Build history of the part. All positions in model axes, mm. A direction names the side the tool comes from. Give positions to 0.01 mm unless a question says otherwise; leave off trailing zeros. Order: outer loops, then holes, each group sorted by start corner. A loop starts at its lowest first (then second) coordinate and runs counter-clockwise, first axis right, second up. Notation, with made-up numbers: M -11.75,-26 L 7.25,-26 A21 ccw 7.25,-13 Z; hole C -4,84 d5. An arc over 180 degrees is marked long. One line per item, written item: value.
from build123d import *

# Parameters (mm, degrees)
F0_W           = 200
F0_H           = 200
F1_DEPTH       = 200
F2_W           = 160
F2_H           = 130
F3_DEPTH       = 160
F5_DEPTH       = 24
F7_R           = 5
F8_DEPTH       = 25
F9_DEPTH       = 25
F9_DEPTH_BACK  = 203.2
F10_DEPTH      = 25
F10_DEPTH_BACK = 215.8


with BuildPart() as f1:
    # F0 (on Top) → F1 (new body)
    with BuildSketch(Plane.XY):
        Rectangle(F0_W, F0_H)
    extrude(amount=F1_DEPTH)

    # F2 (on face) → F3 (cut)
    with BuildSketch(Plane.XZ.offset(100)):
        with Locations((0, 80)):
            Rectangle(F2_W, F2_H)
    extrude(amount=-F3_DEPTH, mode=Mode.SUBTRACT)

    # F4 (on face) → F5 (cut)
    with BuildSketch(Plane.YZ.offset(100)):
        Polygon((-7.5, 67.5), (0, 67.5), (7.5, 67.5), (7.5, 82.5), (-7.5, 82.5), align=None)
    extrude(amount=-F5_DEPTH, mode=Mode.SUBTRACT)

    # F6 (on face) + F7 (on face) → F8 (cut)
    with BuildSketch(Plane(origin=(-100, 0, 0), x_dir=(0, -1, 0), z_dir=(-1, 0, 0))):
        Polygon((-7.5, 67.5), (0, 67.5), (7.5, 67.5), (7.5, 82.5), (-7.5, 82.5), align=None)
    with BuildSketch(Plane.YZ.offset(100)):
        with Locations((70, 9)):
            Circle(F7_R)
        with Locations((-70, 9)):
            Circle(F7_R)
    extrude(amount=-F8_DEPTH, mode=Mode.SUBTRACT)

    # F7 (on face) → F9 (cut, two sides)
    with BuildSketch(Plane.YZ.offset(100)) as f9_sk:
        with Locations((-70, 9)):
            Circle(F7_R)
    extrude(amount=F9_DEPTH, mode=Mode.SUBTRACT)
    extrude(f9_sk.sketch, amount=-F9_DEPTH_BACK, mode=Mode.SUBTRACT)

    # F7 (on face) → F10 (cut, two sides)
    with BuildSketch(Plane.YZ.offset(100)) as f10_sk:
        with Locations((70, 9)):
            Circle(F7_R)
    extrude(amount=F10_DEPTH, mode=Mode.SUBTRACT)
    extrude(f10_sk.sketch, amount=-F10_DEPTH_BACK, mode=Mode.SUBTRACT)


solid = f1.part
1) Saw through at C-C, the plane x = 15.5. Write the cut outline in (y, z), then the cut area to 3 significant figures.
Check values:
outline: M -100,0 L 100,0 L 100,200 L -100,200 L -100,145 L 60,145 L 60,15 L -100,15 Z; hole C -70,9 d10; hole C 70,9 d10
area: 19,000 mm^2
2) Saw through at B-B, the plane z = 9. Write the cut outline in (x, y).
Check values:
outline: M -100,-100 L 100,-100 L 100,-75 L -100,-75 Z; M -100,-65 L 100,-65 L 100,65 L -100,65 Z; M -100,75 L 100,75 L 100,100 L -100,100 Z
3) Drill centre lines: probe 1 along Z at (x, y) = (-3.5, -70); probe 2 along X at (y, z) = (31, 111.5); probe 3 along Z at (x, y) = (-42, 70). Where is each one in solid material? Low to high. Write a range as from..to.
Check values:
probe 1: 0..4, 14..15, 145..200
probe 2: -100..-80, 80..100
probe 3: 0..4, 14..200
4) Saw through at D-D, the plane y = 48.5. Write the cut outline in (x, z).
Check values:
outline: M -100,0 L 100,0 L 100,200 L -100,200 Z; hole M -80,15 L 80,15 L 80,145 L -80,145 Z
5) Mould opens along Z. For faces 1 (the face through (-1, 1, 0)), 2 (the face through (-100, -1, 99)), 3 (the face through (-90, 0, 67.5)) say: released by +Z, released by -Z, zero draft, split by the parting line, or undercut.
Check values:
face 1: released by -Z
face 2: zero draft
face 3: undercut
6) Tool access for faces 4 (the face through (-1, 100, 99)), 5 (the face through (-1, -21, 15)), 6 (the face through (-90, -7.5, 75)): list every direction of +Z, -Z, +X, -X, +Y, -Y with a clear straight run to the whole face (end or side of a thin tool).
Check values:
face 4: +Z, -Z, +X, -X, +Y
face 5: -Y
face 6: +X, -X
7) Saw through at A-A, the plane y = -70. Write the cut outline in (x, z), then the cut area to 3 significant figures.
Check values:
outline: M -100,0 L 100,0 L 100,4 L -100,4 Z; M -100,14 L 100,14 L 100,200 L -100,200 Z; hole M -80,15 L 80,15 L 80,145 L -80,145 Z
area: 17,200 mm^2
